Geometry check sheet. Reference: the model listing, model coordinates, mm. Give positions to 0.01 mm unless a question says otherwise; leave off trailing zeros. Loops run counter-clockwise (first coordinate to the right, second up) from the corner with the lowest first, then second, coordinate; pieces in that order, holes last. Notation, with made-up numbers: (-24.5, 13) - (-5.5, 13) arc R21 ccw to (-5.5, 49) - close; hole circle Ø2 at (25, 25.25). An arc over 180 degrees is marked (long way). One line per question, with ' | ' between items. Start each with the question number.
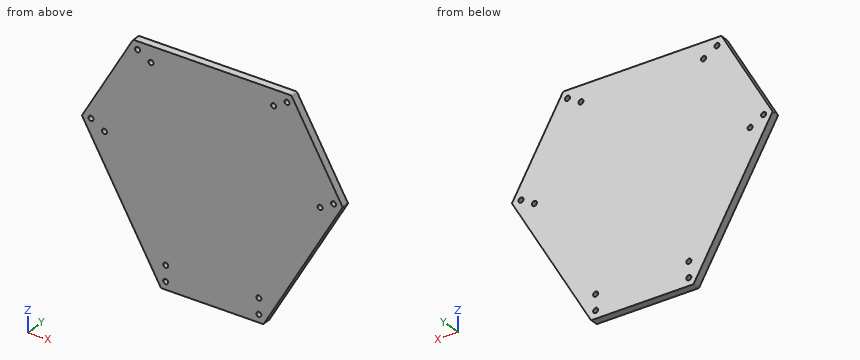
from build123d import *

# Parameters (mm, degrees)
EXTRUDE_1_DEPTH          = 2.5
FILLET_1_R               = 1
SKETCH_3_R               = 1.6
CUT_EXTRUDE_1_DEPTH      = 115.530801874
PATTERN_CIRCULAR_1_COUNT = 3


with BuildPart() as part:
    # Sketch 2 → Extrude 1 (new, symmetric)
    with BuildSketch(Plane(origin=(0, 0, 0), x_dir=(1, 0, 0), z_dir=(0, 1, 0))):
        Polygon((-83.963378955, -10.371161675), (-50.963378955, -67.528838325), (50.963378955, -67.528838325), (83.963378955, -10.371161675), (33, 77.9), (-33, 77.9), align=None)
    extrude(amount=EXTRUDE_1_DEPTH, both=True)

    # Fillet 1
    fillet_1_edges = [part.edges().sort_by_distance(p)[0] for p in [
        (-33, 0, -77.9),
        (33, 0, -77.9),
        (83.963378955, 0, 10.371161675),
        (50.963378955, 0, 67.528838325),
        (-50.963378955, 0, 67.528838325),
        (-83.963378955, 0, 10.371161675),
    ]]
    fillet(fillet_1_edges, radius=FILLET_1_R)

    # Sketch 3 → Cut-Extrude 1 (cut, symmetric)
    with BuildSketch(Plane(origin=(0, 2.5, 0), x_dir=(1, 0, 0), z_dir=(0, 1, 0))):
        with Locations(Location((-30, 72.9, 0), (0, 0, 270))):
            Circle(SKETCH_3_R)
        with Locations(Location((-30, 62.9, 0), (0, 0, 270))):
            Circle(SKETCH_3_R)
        with Locations(Location((30, 62.9, 0), (0, 0, 270))):
            Circle(SKETCH_3_R)
        with Locations(Location((30, 72.9, 0), (0, 0, 270))):
            Circle(SKETCH_3_R)
    cut_extrude_1 = extrude(amount=CUT_EXTRUDE_1_DEPTH, both=True, mode=Mode.SUBTRACT)

    # Pattern Circular 1: Cut-Extrude 1 ×3 about axis
    pattern_circular_1_axis = Axis((0, 0, 0), (0, 1, 0))
    for i in range(1, PATTERN_CIRCULAR_1_COUNT):
        add(cut_extrude_1.rotate(pattern_circular_1_axis, i * 360 / PATTERN_CIRCULAR_1_COUNT), mode=Mode.SUBTRACT)


solid = part.part
(1) Depth check by flat-ended pin: pin 1 Ø3.5 at (x, z) = (39.47, 57.43) entering from -Y; pin 2 Ø2.5 at (x, z) = (-48.13, 62.43) entering from +Y. Enter the tip coordinate at first touch or a pass-through.
(2) Section check C-C, the plane z = -14. Record the boundary of the cut face in (x, y).
(3) Section check A-A, the plane y = 1.25. Count the separate pieces of the cut face and the enclosed holes in it, and give its area (3 significant figures).
(4) Section check B-B, the plane z = -33.5. Record the boundary of the cut face in (x, y).
(5) Material ranges on line 1 (X direction, y = -0.8, z = -72.9); line 2 (X direction, y = 0.5, z = -62.9); line 3 (Z direction, x = 59.5, y = -1.7), recorded low to high.
Numbers:
1) pin 1: y = -2.5 | pin 2: through
2) outline: (-69.89, -2.5) - (69.89, -2.5) - (69.89, 2.5) - (-69.89, 2.5) - close
3) separate pieces: 1 | enclosed holes: 12 | area: 17,900 mm^2
4) outline: (-58.63, -2.5) - (58.63, -2.5) - (58.63, 2.5) - (-58.63, 2.5) - close
5) line 1: -35.89 to -31.6, -28.4 to 28.4, 31.6 to 35.89 | line 2: -41.66 to -31.6, -28.4 to 28.4, 31.6 to 41.66 | line 3: -32 to 52.74
